Could you check a few things on this model? Use its own coordinates, in mm. A direction names the side the tool comes from. Give positions to 0.01 mm unless a question says otherwise; leave off trailing zeros. Loops run counter-clockwise (first coordinate to the right, second up) from the corner with the lowest first, then second, coordinate; pieces in that order, holes last. Notation, with made-up numbers: (-13, 28.25) - (40, 28.25) arc R5 cw to (40, 32.25) - close; hole circle Ø8 at (71.5, 14). An arc over 180 degrees is marked (long way). Write each question's results on one line, items separated by ' | '. Start each with the question number.
```python
from build123d import *

# Parameters (mm, degrees)
SKETCH1_W                = 6
SKETCH1_H                = 8
BOSS_EXTRUDE1_DEPTH      = 3
SKETCH3_W                = 5
SKETCH3_H                = 6
BOSS_EXTRUDE3_DEPTH      = 6
SKETCH4_R                = 2
CUT_EXTRUDE1_DEPTH       = 53.971690553
BOSS_EXTRUDE4_DEPTH      = 6
BOSS_EXTRUDE4_DEPTH_BACK = 3
SKETCH5_W                = 6
SKETCH5_H                = 8
SKETCH6_R                = 2
CUT_EXTRUDE2_DEPTH       = 6
SKETCH7_W                = 3
SKETCH7_H                = 1
CUT_EXTRUDE3_DEPTH       = 10
CUT_EXTRUDE4_DEPTH       = 10
CUT_EXTRUDE4_DEPTH_BACK  = 10
SKETCH8_W                = 3
SKETCH8_H                = 1
SKETCH8_W_2              = 20.55867335
SKETCH8_H_2              = 13.11372747


with BuildPart() as part:
    # Sketch1 → Boss-Extrude1 (new body)
    with BuildSketch(Plane(origin=(0, 0, 0), x_dir=(1, 0, 0), z_dir=(0, 1, 0))):
        Polygon((3, 15), (25, 15), (25, -15), (-25, -15), (-25, 15), (-3, 15), align=None)
        with Locations((0, 9)):
            Rectangle(SKETCH1_W, SKETCH1_H, mode=Mode.SUBTRACT)
    extrude(amount=BOSS_EXTRUDE1_DEPTH)

    # Sketch3 → Boss-Extrude3 (add)
    with BuildSketch(Plane(origin=(0, 3, 0), x_dir=(1, 0, 0), z_dir=(0, 1, 0))):
        with Locations((-22.5, -2)):
            Rectangle(SKETCH3_W, SKETCH3_H)
        with Locations((22.5, -2)):
            Rectangle(SKETCH3_W, SKETCH3_H)
    extrude(amount=BOSS_EXTRUDE3_DEPTH)

    # Sketch4 → Cut-Extrude1 (cut, through all)
    with BuildSketch(Plane.ZY.offset(25)):
        with Locations((2, 6)):
            Circle(SKETCH4_R)
    extrude(amount=-CUT_EXTRUDE1_DEPTH, mode=Mode.SUBTRACT)

    # Sketch5 → Boss-Extrude4 (add, two sides: drawn at the far end of the back side and taken through both)
    with BuildSketch(Plane(origin=(0, 3, 0), x_dir=(-1, 0, 0), z_dir=(0, 1, 0)).offset(-BOSS_EXTRUDE4_DEPTH_BACK)):
        with Locations((0, -9)):
            Rectangle(SKETCH5_W, SKETCH5_H)
    extrude(amount=BOSS_EXTRUDE4_DEPTH + BOSS_EXTRUDE4_DEPTH_BACK)

    # Sketch6 → Cut-Extrude2 (cut)
    with BuildSketch(Plane.ZY.offset(3)):
        with Locations((-9, 6)):
            Circle(SKETCH6_R)
    extrude(amount=-CUT_EXTRUDE2_DEPTH, mode=Mode.SUBTRACT)

    # Sketch7 → Cut-Extrude3 (cut)
    with BuildSketch(Plane(origin=(0, 3, 0), x_dir=(-1, 0, 0), z_dir=(0, 1, 0))):
        with Locations((14, -0.5)):
            Rectangle(SKETCH7_W, SKETCH7_H)
        with Locations((-14, -0.5)):
            Rectangle(SKETCH7_W, SKETCH7_H)
        with Locations((-14, 4.5)):
            Rectangle(SKETCH7_W, SKETCH7_H)
        with Locations((14, 4.5)):
            Rectangle(SKETCH7_W, SKETCH7_H)
    extrude(amount=-CUT_EXTRUDE3_DEPTH, mode=Mode.SUBTRACT)

    # Sketch8 → Cut-Extrude4 (cut, two sides: drawn at the far end of the back side and taken through both)
    with BuildSketch(Plane(origin=(0, 3, 0), x_dir=(1, 0, 0), z_dir=(0, 1, 0)).offset(-CUT_EXTRUDE4_DEPTH_BACK)):
        with Locations((-13.5, 11.5)):
            Rectangle(SKETCH8_W, SKETCH8_H)
        with Locations((13.5, 11.5)):
            Rectangle(SKETCH8_W, SKETCH8_H)
        with Locations((-13.5, 6.5)):
            Rectangle(SKETCH8_W, SKETCH8_H)
        with Locations((13.5, 6.5)):
            Rectangle(SKETCH8_W, SKETCH8_H)
        with Locations((0, 9)):
            Rectangle(SKETCH8_W_2, SKETCH8_H_2)
    extrude(amount=CUT_EXTRUDE4_DEPTH + CUT_EXTRUDE4_DEPTH_BACK, mode=Mode.SUBTRACT)


solid = part.part
```
Q1. I need wall thicknesses on L1, parallel to X at y = 1.5, z = -10; L2, parallel to Y at x = 23.15, z = 2; L3, parallel to X at y = 8.75, z = 0.5. Which ranges of each line are inside material? Lowest first, please. Write a range as from..to.
Q2. I want a section at D-D, the plane z = -12.5. List the corners of the cut face in (x, y) for me, then the cut area to 3 significant figures.
Q3. If we mould it in two halves opening along Z, with no side actions, what happens to faces 1 (the face through (0, 1, -2.443)), 2 (the face through (0, 3, 0)), 3 (the face through (12, 1.5, -11.5))? For each: +Z half, -Z half, draft (parallel to the pull), parting line (faces both ways), or undercut.
Q4. Which directions (+Z, -Z, +X, -X, +Y, -Y) give clear straight access to the entire face, cutting with the end or side of a thin tool? Please do faces 4 (the face through (-18, 1, -15)), 5 (the face through (-14, 2, 4)), 6 (the face through (-23, 9, 2)), 7 (the face through (-23, 6, -1)), 8 (the face through (22, 6, 5)).
Q5. I want a section at A-A, the plane y = 8.5. List the corners of the cut face in (x, z) for me.
Q6. I want a section at C-C, the plane y = 6. List the corners of the cut face in (x, z) for me, then the cut area to 3 significant figures.
Q7. I'm going to push a flat-ended pin straight in: pin 1 Ø10 at (x, z) = (-13, 11) entering from +Y. Where does the tip first touch, or does it pass through?
Q8. I want a section at B-B, the plane z = 2. List the corners of the cut face in (x, y) for me, then the cut area to 3 significant figures.
Conclusion:
1) L1: -25..-10.28, 10.28..25 | L2: 0..4, 8..9 | L3: -25..-20, 20..25
2) outline: (-25, 0) - (-10.28, 0) - (-10.28, 3) - (-25, 3) - close; (10.28, 0) - (25, 0) - (25, 3) - (10.28, 3) - close | area: 88.3 mm^2
3) face 1: -Z half | face 2: draft | face 3: undercut
4) face 4: -Z, +X, -X, +Y, -Y | face 5: +Y, -Y | face 6: +Z, -Z, +X, -X, +Y | face 7: -Z, +X, -X, +Y | face 8: +Z, +X, -X, +Y
5) outline: (-25, -1) - (-20, -1) - (-20, 5) - (-25, 5) - close; (20, -1) - (25, -1) - (25, 5) - (20, 5) - close
6) outline: (-25, -1) - (-20, -1) - (-20, 0) - (-25, 0) - close; (-25, 4) - (-20, 4) - (-20, 5) - (-25, 5) - close; (20, -1) - (25, -1) - (25, 0) - (20, 0) - close; (20, 4) - (25, 4) - (25, 5) - (20, 5) - close | area: 20.0 mm^2
7) pin 1: y = 3
8) outline: (-25, 0) - (25, 0) - (25, 4) - (20, 4) - (20, 3) - (-20, 3) - (-20, 4) - (-25, 4) - close; (-25, 8) - (-20, 8) - (-20, 9) - (-25, 9) - close; (20, 8) - (25, 8) - (25, 9) - (20, 9) - close | area: 170 mm^2
